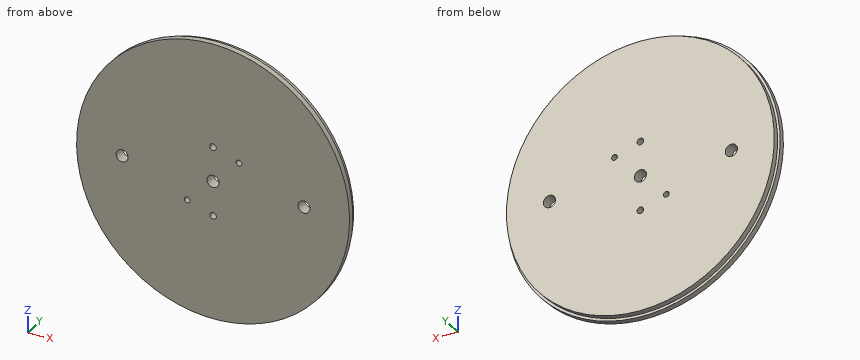
from build123d import *

# Parameters (mm, degrees)
SKETCH1_R                    = 76.2
BOSS_EXTRUDE1_DEPTH          = 1.5875
SKETCH2_R                    = 74.7776
BOSS_EXTRUDE2_DEPTH          = 3.175
SKETCH3_R                    = 3.3782
CUT_EXTRUDE1_DEPTH           = 108.95
F_27_0_144_DIAMETER_HOLE1_D  = 3.6576
F_1_8_0_125_DIAMETER_HOLE1_D = 3.175


with BuildPart() as part:
    # Sketch1 → Boss-Extrude1 (new, symmetric)
    with BuildSketch(Plane(origin=(0, 0, 0), x_dir=(1, 0, 0), z_dir=(0, 1, 0))):
        with Locations(Location((0, 0, 0), (0, 0, 270))):
            Circle(SKETCH1_R)
    extrude(amount=BOSS_EXTRUDE1_DEPTH, both=True)

    # Sketch2 → Boss-Extrude2 (add)
    with BuildSketch(Plane(origin=(0, 1.5875, 0), x_dir=(1, 0, 0), z_dir=(0, 1, 0))):
        with Locations(Location((0, 0, 0), (0, 0, 270))):
            Circle(SKETCH2_R)
    extrude(amount=BOSS_EXTRUDE2_DEPTH)

    # Sketch3 → Cut-Extrude1 (cut, through all)
    with BuildSketch(Plane.XZ.offset(1.5875)):
        with Locations(Location((50.8, 0, 0), (0, 0, 270))):
            Circle(SKETCH3_R)
        with Locations(Location((-50.8, 0, 0), (0, 0, 270))):
            Circle(SKETCH3_R)
        with Locations(Location((0, 0, 0), (0, 0, 270))):
            Circle(SKETCH3_R)
    extrude(amount=-CUT_EXTRUDE1_DEPTH, mode=Mode.SUBTRACT)

    # #27 (0.144) Diameter Hole1 (through all)
    with Locations(Plane(origin=(0, -1.5875, 0), x_dir=(-1, 0, 0), z_dir=(0, -1, 0))):
        with Locations((0, 19.05), (0, -19.05)):
            Hole(F_27_0_144_DIAMETER_HOLE1_D / 2)

    # 1/8 (0.125) Diameter Hole1 (through all)
    with Locations(Plane(origin=(0, -1.5875, 0), x_dir=(-1, 0, 0), z_dir=(0, -1, 0))):
        with Locations((14.469766177, 14.266333333), (-14.469766177, -14.266333333)):
            Hole(F_1_8_0_125_DIAMETER_HOLE1_D / 2)


solid = part.part
Design review of the part built by this model. Coordinates are the model's own, in mm. Round coordinates to 2 decimals unless told otherwise and drop trailing zeros. Write each loop counter-clockwise with the first axis right and the second up, starting at its lowest first coordinate (ties: lowest second). Pieces come first, ordered by that corner, then holes.
Item 1: For pin 1 Ø2 at (x, y) = (22.5, 3) entering from -Z; pin 2 Ø1 at (x, y) = (14, 2) entering from +Z; pin 3 Ø3 at (y, z) = (1, 30.5) entering from -X, all flat-tipped, find the tip position at first contact; note any pin that passes through.
Item 2: Wall thickness on L1, parallel to X at y = 0.75, z = 0.5; L2, parallel to X at y = 0.5, z = 0; L3, parallel to X at y = 2, z = -19.05: over which ranges is each line inside the solid? List them lowest first.
Item 3: Consider section C-C on x = -50.8. Give the boundary of the cut face in (y, z).
Item 4: Consider section B-B on x = 0. Give the boundary of the cut face in (y, z), and give its area (3 significant figures).
Item 5: Consider section A-A on z = 0. Give the boundary of the cut face in (x, y).
Item 6: Consider section D-D on y = 3.75. Count the separate pieces of the cut face and the enclosed holes in it, and give its area (3 significant figures).
Check values:
1. pin 1: stops at z = -71.62
1. pin 2: stops at z = 74.96
1. pin 3: stops at x = -70.47
2. L1: x = -76.2 to -54.14, -47.46 to -3.34, 3.34 to 47.46, 54.14 to 76.2
2. L2: x = -76.2 to -54.18, -47.42 to -3.38, 3.38 to 47.42, 54.18 to 76.2
2. L3: x = -72.31 to -1.83, 1.83 to 72.31
3. outline: (-1.59, -56.8) - (1.59, -56.8) - (1.59, -54.87) - (4.76, -54.87) - (4.76, -3.38) - (-1.59, -3.38) - close; (-1.59, 3.38) - (4.76, 3.38) - (4.76, 54.87) - (1.59, 54.87) - (1.59, 56.8) - (-1.59, 56.8) - close
4. outline: (-1.59, -76.2) - (1.59, -76.2) - (1.59, -74.78) - (4.76, -74.78) - (4.76, -20.88) - (-1.59, -20.88) - close; (-1.59, -17.22) - (4.76, -17.22) - (4.76, -3.38) - (-1.59, -3.38) - close; (-1.59, 3.38) - (4.76, 3.38) - (4.76, 17.22) - (-1.59, 17.22) - close; (-1.59, 20.88) - (4.76, 20.88) - (4.76, 74.78) - (1.59, 74.78) - (1.59, 76.2) - (-1.59, 76.2) - close
4. area: 869 mm2
5. outline: (-76.2, -1.59) - (-54.18, -1.59) - (-54.18, 4.76) - (-74.78, 4.76) - (-74.78, 1.59) - (-76.2, 1.59) - close; (-47.42, -1.59) - (-3.38, -1.59) - (-3.38, 4.76) - (-47.42, 4.76) - close; (3.38, -1.59) - (47.42, -1.59) - (47.42, 4.76) - (3.38, 4.76) - close; (54.18, -1.59) - (76.2, -1.59) - (76.2, 1.59) - (74.78, 1.59) - (74.78, 4.76) - (54.18, 4.76) - close
6. separate pieces: 1
6. enclosed holes: 7
6. area: 17,400 mm2
